The listing builds one solid part. Answer for the finished solid, in the listing's coordinates (mm). Face numbers are marked on the shaded views. A direction names the side the tool comes from. Round coordinates to 2 decimals unless told otherwise and drop trailing zeros. Write each loop counter-clockwise with the first axis right and the second up, starting at its lowest first coordinate (ties: lowest second). Pieces come first, ordered by that corner, then holes. Notation, with made-up numbers: (32.25, 3) - (80.25, 3) arc R16 cw to (80.25, 17) - close; hole circle Ø11 at (38.5, 88). An arc over 180 degrees is marked (long way). Answer in a Markdown table with one row per item.
from build123d import *

# Parameters (mm, degrees)
SKETCH4_R               = 22.225
BOSS_EXTRUDE1_DEPTH     = 59.436
SKETCH5_W               = 2.54
SKETCH5_H               = 2.54
SKETCH6_R               = 17.78
CUT_EXTRUDE1_DEPTH      = 51.816
CUT_EXTRUDE3_DEPTH      = 68.23495628
CUT_EXTRUDE3_DEPTH_BACK = 68.23495628
CUT_EXTRUDE5_REACH      = 77.768
CUT_EXTRUDE5_END_RADIUS = 22.225
SKETCH12_W              = 22.352
SKETCH12_H              = 19.05
SKETCH13_R              = 6.35
CUT_EXTRUDE6_DEPTH      = 5.842


with BuildPart() as part:
    # Sketch4 → Boss-Extrude1 (new body)
    with BuildSketch(Plane(origin=(0, 0, 0), x_dir=(1, 0, 0), z_dir=(0, 1, 0))):
        with Locations(Location((0, 0, 0), (0, 0, 270))):
            Circle(SKETCH4_R)
    extrude(amount=-BOSS_EXTRUDE1_DEPTH)

    # Sketch5 → Cut-Revolve1 (revolve, cut)
    with BuildSketch(Plane.XY, mode=Mode.PRIVATE) as cut_revolve1_sk:
        with Locations((20.955, -8.89)):
            Rectangle(SKETCH5_W, SKETCH5_H)
        with Locations((20.955, -13.97)):
            Rectangle(SKETCH5_W, SKETCH5_H)
        with Locations((20.955, -19.05)):
            Rectangle(SKETCH5_W, SKETCH5_H)
    revolve(cut_revolve1_sk.sketch.rotate(Axis((0, 26.260199794, 0), (0, -1, 0)), 90), axis=Axis((0, 26.260199794, 0), (0, -1, 0)), mode=Mode.SUBTRACT)

    # Sketch6 → Cut-Extrude1 (cut)
    with BuildSketch(Plane.XZ.offset(59.436)):
        with Locations(Location((0, 0, 0), (0, 0, 270))):
            Circle(SKETCH6_R)
    extrude(amount=-CUT_EXTRUDE1_DEPTH, mode=Mode.SUBTRACT)

    # Sketch7 → Cut-Extrude3 (cut, two sides: drawn at the far end of the back side and taken through both)
    with BuildSketch(Plane.XY.offset(-CUT_EXTRUDE3_DEPTH_BACK)):
        with BuildLine():
            Line((22.225, -59.436), (22.225, -51.816))
            Line((22.225, -51.816), (13.459535823, -51.816))
            ThreePointArc((13.459535823, -51.816), (11.659833258, -52.274635573), (10.289790639, -53.52853315))
            Line((10.289790639, -53.52853315), (6.35, -59.436))
            Line((6.35, -59.436), (22.225, -59.436))
        make_face()
        with BuildLine():
            Line((-22.225, -59.436), (-6.35, -59.436))
            Line((-6.35, -59.436), (-10.289790639, -53.52853315))
            ThreePointArc((-10.289790639, -53.52853315), (-11.659833258, -52.274635573), (-13.459535823, -51.816))
            Line((-13.459535823, -51.816), (-22.225, -51.816))
            Line((-22.225, -51.816), (-22.225, -59.436))
        make_face()
    extrude(amount=CUT_EXTRUDE3_DEPTH + CUT_EXTRUDE3_DEPTH_BACK, mode=Mode.SUBTRACT)

    # Cut-Extrude5: up to this cylinder (the profile starts inside it)
    cut_extrude5_end = Plane(origin=(0, -34.178757, 0), z_dir=(0, 1, 0)) * Cylinder(CUT_EXTRUDE5_END_RADIUS, 200.986, mode=Mode.PRIVATE)
    # Sketch12 → Cut-Extrude5 (cut, up to the surface)
    with BuildSketch(Plane.XY.offset(19.177), mode=Mode.PRIVATE) as cut_extrude5_sk1:
        with Locations((0, -34.17875674)):
            Rectangle(SKETCH12_W, SKETCH12_H)
    cut_extrude5_tool1 = extrude(cut_extrude5_sk1.sketch, amount=CUT_EXTRUDE5_REACH, mode=Mode.PRIVATE) & cut_extrude5_end
    cut_extrude5 = cut_extrude5_tool1.solids().sort_by_distance((0, -34.178757, 19.177))[0]
    add(cut_extrude5, mode=Mode.SUBTRACT)

    # Sketch13 → Cut-Extrude6 (cut)
    with BuildSketch(Plane.XY.offset(19.177)):
        with Locations((0, -34.17875674)):
            Circle(SKETCH13_R)
    cut_extrude6 = extrude(amount=-CUT_EXTRUDE6_DEPTH, mode=Mode.SUBTRACT)

    # Mirror1: Cut-Extrude5, Cut-Extrude6 across plane
    add(cut_extrude5.mirror(Plane.XY), mode=Mode.SUBTRACT)
    add(cut_extrude6.mirror(Plane.XY), mode=Mode.SUBTRACT)

    # Sketch16 → Cut-Revolve2 (revolve, cut)
    with BuildSketch(Plane.XY, mode=Mode.PRIVATE) as cut_revolve2_sk:
        with BuildLine():
            Line((0, 0), (0, -1.27))
            ThreePointArc((0, -1.27), (6.387986381, -0.951711763), (12.712693656, 0))
            Line((12.712693656, 0), (0, 0))
        make_face()
    revolve(cut_revolve2_sk.sketch.rotate(Axis((0, 62.992, 0), (0, -1, 0)), 180), axis=Axis((0, 62.992, 0), (0, -1, 0)), mode=Mode.SUBTRACT)


solid = part.part
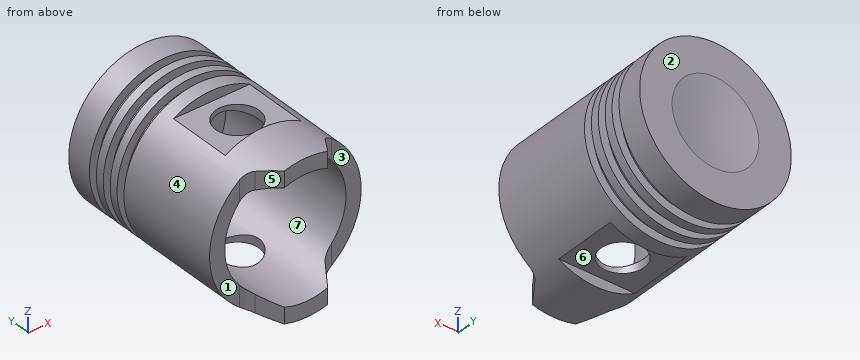
(1) Flat-ended cylindrical pins translate along their axes: pin 1 (16.5 mm diameter, centred on x = 0, y = -34.18, fed in from +Z); pin 2 (9.5 mm diameter, centred on x = 17.5, z = -0.5, fed in from -Y); pin 3 (1.5 mm diameter, centred on x = -2, z = 1, fed in from -Y). Find the tip coordinate at first contact, or state that the pin passes through.
Checked values:
| item | result |
|---|---|
| pin 1 | stops at z = 19.18 |
| pin 2 | stops at y = -51.82 |
| pin 3 | stops at y = -7.62 |
(2) Section B-B (x = 0) is taken. State how many separate pieces and enclosed holes the cut face has, and give its area (3 significant figures).
Checked values:
| item | result |
|---|---|
| separate pieces | 3 |
| enclosed holes | 0 |
| area | 587 mm2 |
(3) For the marked faces 1, 2, 3 and 4, determine the directions among +Z, -Z, +X, -X, +Y, -Y from which every point of the face is accessible in a straight line to the end or side of a thin tool.
Checked values:
| item | result |
|---|---|
| face 1 | +Z, -Z, -X, -Y |
| face 2 | +Z, -Z, +X, -X, +Y |
| face 3 | +Z, -Z, +X, -Y |
| face 4 | +Y, -Y |
(4) Section C-C (y = -56) is taken. Give the vertices of the cut face in (x, z) (3 decimals), and give its area (3 significant figures).
Checked values:
| item | result |
|---|---|
| outline | (-8.642, -20.476) arc R22.225 ccw to (8.642, -20.476) - (8.642, -15.539) arc R17.78 cw to (-8.642, -15.539) - close; (-8.642, 15.539) arc R17.78 cw to (8.642, 15.539) - (8.642, 20.476) arc R22.225 ccw to (-8.642, 20.476) - close |
| area | 159 mm2 |
(5) For a pull along Z with two mould halves and no side action, classify the marked faces 5, 6 and 7 as pulls with the +Z half, pulls with the -Z half, needs draft (parallel to the pull), parting line crosses it, or undercut.
Checked values:
| item | result |
|---|---|
| face 5 | needs draft |
| face 6 | pulls with the -Z half |
| face 7 | undercut |
(6) Section A-A (y = -19) is taken. Give the vertices of the cut face in (x, z) (3 decimals).
Checked values:
| item | result |
|---|---|
| outline | circle Ø39.37 at (0, 0); hole circle Ø35.56 at (0, 0) |
(7) Find the intervals of material crossed by line 1 (Y direction, x = 19, z = 8); line 2 (Y direction, x = 0, z = -18.1); line 3 (X direction, y = -31, z = 0) (3 decimals), in increasing order.
Checked values:
| item | result |
|---|---|
| line 1 | y = -51.82 to -20.32, -17.78 to -15.24, -12.7 to -10.16, -7.62 to 0 |
| line 2 | y = -59.44 to -40.53, -27.83 to 0 |
| line 3 | x = -22.225 to -17.78, 17.78 to 22.225 |
